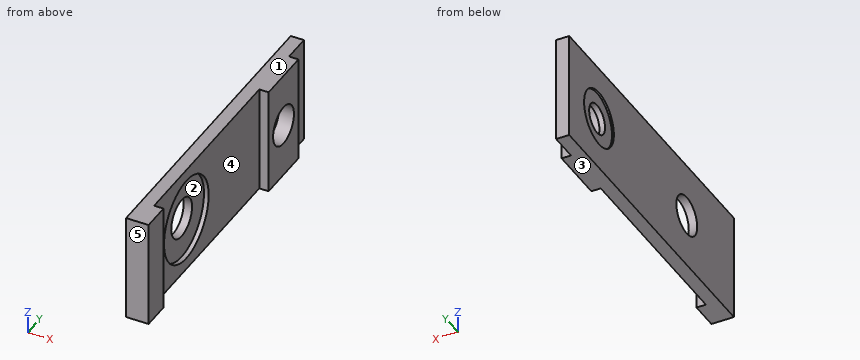
from build123d import *

# Parameters (mm, degrees)
SALIENTE_EXTRUIR1_DEPTH = 11.5
CORTAR_EXTRUIR1_START   = -2.4
CROQUIS2_R              = 2.1
CORTAR_EXTRUIR1_DEPTH   = 2.4
CROQUIS3_R              = 4.5
CORTAR_EXTRUIR2_DEPTH   = 0.5
CROQUIS4_R              = 3
CORTAR_EXTRUIR3_DEPTH   = 0.2
CROQUIS5_R              = 2.1
CROQUIS5_R_2            = 1.6
SALIENTE_EXTRUIR2_DEPTH = 0.6


with BuildPart() as part:
    # Croquis1 → Saliente-Extruir1 (new body)
    with BuildSketch(Plane.XY):
        Polygon((-89.253382482, -13.336480186), (-89.253382482, 19.863519814), (-87.853382482, 19.863519814), (-87.853382482, 16.863519814), (-86.853382482, 16.863519814), (-86.853382482, 10.863519814), (-87.853382482, 10.863519814), (-87.853382482, -10.336480186), (-86.853382482, -10.336480186), (-86.853382482, -13.336480186), align=None)
    extrude(amount=SALIENTE_EXTRUIR1_DEPTH)

    # Croquis2 → Cortar-Extruir1 (cut)
    with BuildSketch(Plane(origin=(-86.853382482, 0, 0), x_dir=(0, 0, -1), z_dir=(1, 0, 0)).offset(CORTAR_EXTRUIR1_START)):
        with Locations((-5.75, 13.863519814)):
            Circle(CROQUIS2_R)
        with Locations((-5.75, -3.836480186)):
            Circle(CROQUIS2_R)
    extrude(amount=CORTAR_EXTRUIR1_DEPTH, mode=Mode.SUBTRACT)

    # Croquis3 → Cortar-Extruir2 (cut)
    with BuildSketch(Plane(origin=(-87.853382482, 0, 0), x_dir=(0, 0, -1), z_dir=(1, 0, 0))):
        with Locations((-5.75, -3.836480186)):
            Circle(CROQUIS3_R)
    extrude(amount=-CORTAR_EXTRUIR2_DEPTH, mode=Mode.SUBTRACT)

    # Croquis4 → Cortar-Extruir3 (cut)
    with BuildSketch(Plane.ZY.offset(89.253382482)):
        with Locations((5.75, 13.863519814)):
            Circle(CROQUIS4_R)
    extrude(amount=-CORTAR_EXTRUIR3_DEPTH, mode=Mode.SUBTRACT)

    # Croquis5 → Saliente-Extruir2 (add)
    with BuildSketch(Plane.ZY.offset(89.053382482)):
        with Locations((5.75, 13.863519814)):
            Circle(CROQUIS5_R)
        with Locations((5.75, 13.863519814)):
            Circle(CROQUIS5_R_2, mode=Mode.SUBTRACT)
    extrude(amount=-SALIENTE_EXTRUIR2_DEPTH)


solid = part.part
Verification items for the finished model (mm, model axes). Face numbers are marked on the shaded views. A direction names the side the tool comes from. Coordinates: 2 decimals unless noted, no trailing zeros. Loops run counter-clockwise (first coordinate to the right, second up) from the corner with the lowest first, then second, coordinate; pieces in that order, holes last. Notation, with made-up numbers: (-36.75, 24.25) -> (-20.75, 24.25) arc R8 ccw to (-20.75, 30.25) -> close; hole circle Ø5 at (18, -13). An arc over 180 degrees is marked (long way). Answer as a JSON object with one key per item and string values. Group by question number.
Item 1: Sectioned sample at D-D on y = 1. Record the boundary of the cut face in (x, z), plus the area to 3 significant figures.
Item 2: Mould release check, pull along Z, two halves, no side actions. Record for the marked faces 1, 2 and 3: +Z half, -Z half, draft (parallel to the pull), parting line (faces both ways), or undercut.
Item 3: Tool access check on the marked faces 4 and 5. Record the directions out of +Z, -Z, +X, -X, +Y, -Y that give a thin tool (end or side, any length) a straight path to the whole face; none if there is none.
Item 4: Sectioned sample at C-C on y = -5.5. Record the boundary of the cut face in (x, z).
Item 5: Scan lines: probe 1 along Y at (x, z) = (-89.1, 5.75); probe 2 along Y at (x, z) = (-88.8, 5.75); probe 3 along Y at (x, z) = (-87.2, 8). Record each from-to range of solid material in increasing order.
Item 6: Depth check by flat-ended pin: pin 1 (4 mm diameter, centred on y = -3.84, z = 5.75, fed in from +X); pin 2 (2 mm diameter, centred on y = 4, z = 7.5, fed in from +X); pin 3 (2.5 mm diameter, centred on y = -6, z = 5.5, fed in from +X). Enter the tip coordinate at first touch or a pass-through.
Item 7: Sectioned sample at A-A on z = 5.75. State how many separate pieces and enclosed holes the cut face has, plus the area to 3 significant figures.
Item 8: Sectioned sample at B-B on x = -87.5. Record the boundary of the cut face in (y, z), plus the area to 3 significant figures.
Evaluation:
{
 "1": {"outline": "(-89.25, 0) -> (-87.85, 0) -> (-87.85, 11.5) -> (-89.25, 11.5) -> close", "area": "16.1 mm²"},
 "2": {"face 1": "+Z half", "face 2": "undercut", "face 3": "-Z half"},
 "3": {"face 4": "+Z, -Z, +X", "face 5": "+Z, -Z, +X, -X, -Y"},
 "4": {"outline": "(-89.25, 0) -> (-87.85, 0) -> (-87.85, 1.57) -> (-88.35, 1.57) -> (-88.35, 4.47) -> (-89.25, 4.47) -> close; (-89.25, 7.03) -> (-88.35, 7.03) -> (-88.35, 9.93) -> (-87.85, 9.93) -> (-87.85, 11.5) -> (-89.25, 11.5) -> close"},
 "5": {"probe 1": "y = -13.34 to -5.94, -1.74 to 10.86, 16.86 to 19.86", "probe 2": "y = -13.34 to -5.94, -1.74 to 12.26, 15.46 to 19.86", "probe 3": "y = -13.34 to -10.34, 10.86 to 16.86"},
 "6": {"pin 1": "passes through", "pin 2": "stops at x = -87.85", "pin 3": "stops at x = -88.35"},
 "7": {"separate pieces": "3", "enclosed holes": "0", "area": "37.4 mm²"},
 "8": {"outline": "(-13.34, 0) -> (-10.34, 0) -> (-10.34, 11.5) -> (-13.34, 11.5) -> close; (10.86, 0) -> (16.86, 0) -> (16.86, 11.5) -> (10.86, 11.5) -> close; hole circle Ø4.2 at (13.86, 5.75)", "area": "89.6 mm²"}
}
